Autodesk Fusion 360 part; units mm, degrees
sketch "スケッチ1" plane through (0, 0, 0) normal (0, 0, 1) x (1, 0, 0)
  circle A0 centre (0, 0) radius 10.55
  dimension "d1" = 21.1
extrude "押し出し1" add sketch "スケッチ1" along normal blind 2
sketch "スケッチ2" plane through (0, 0, 2) normal (0, 0, 1) x (-1, 0, 0)
  circle A0 centre (0, 0) radius 10.55
  circle A1 centre (0, 0) radius 8.5
  dimension "d4" = 17
extrude "押し出し2" add sketch "スケッチ2" along normal blind 3.2 contours A1
sketch "スケッチ3" plane through (0, 0, 5.2) normal (0, 0, 1) x (-1, 0, 0)
  circle A0 centre (0, 0) radius 8.5
  circle A1 centre (0, 0) radius 10.55
extrude "押し出し3" add sketch "スケッチ3" along normal blind 2 contours A0 | A1
sketch "スケッチ4" plane through (0, 0, 7.2) normal (0, 0, 1) x (-1, 0, 0)
  line L0 (10.5233, -0.75) -> (-10.5233, -0.75)
  line L1 (10.5233, 0.75) -> (-10.5233, 0.75)
  circle A0 centre (0, 0) radius 10.55
  dimension "d24" = 0.75
  dimension "d25" = 0.75
extrude "押し出し7" add sketch "スケッチ4" along normal blind 30 contours L0 L1 A0
sketch "スケッチ5" plane through (0, -0.75, 0) normal (0, -1, 0) x (1, 0, 0)
  line L0 (-10.4732, 7.2) -> (10.4732, 7.2)
  line L1 (10.5, 7.2) -> (10.5, 37.2)
  line L2 (10.5, 37.2) -> (-10.5, 37.2)
  line L3 (-10.5, 37.2) -> (-10.5, 7.2)
  circle A0 centre (0, 34.2) radius 1.625
  line L4 (0, 34.2) -> (0, 37.2) construction
  line L5 (10.4732, 7.2) -> (10.5, 7.2)
  line L6 (-10.5, 7.2) -> (-10.4732, 7.2)
  line L7 (-10.5233, 7.2) -> (10.5233, 7.2)
  line L8 (10.5233, 7.2) -> (10.5233, 37.2)
  line L9 (10.5233, 37.2) -> (-10.5233, 37.2)
  line L10 (-10.5233, 37.2) -> (-10.5233, 7.2)
  dimension "d13" = 3.25
  dimension "d14" = 3
extrude "押し出し8" cut sketch "スケッチ5" against normal up to surface (1.5 mm away) contours A0
sketch "スケッチ8" plane through (0, 0, 7.2) normal (0, 0, 1) x (-1, 0, 0)
  line L0 (-10.5233, 0.75) -> (10.5233, 0.75)
  arc A0 (10.5233, 0.75) -> (-10.5233, 0.75) centre (0, 0) ccw
  line L1 (0.75, -10.5233) -> (0.75, 10.5233)
  line L2 (-0.75, -10.5233) -> (-0.75, 10.5233)
  arc A1 (-10.5233, -0.75) -> (10.5233, -0.75) centre (0, 0) ccw
  dimension "d30" = 0.75
  dimension "d31" = 0.75
extrude "押し出し9" add sketch "スケッチ8" along normal blind 20 contours L0 A0 L1 L2 | L0 L1 L2 A1
Work out the finished part from the listing and answer in its coordinate system (mm). A direction names the side the tool comes from. Coordinates: 2 decimals unless noted, no trailing zeros. Order: outer loops, then holes, each group sorted by start corner. A loop starts at its lowest first (then second) coordinate and runs counter-clockwise, first axis right, second up. Notation, with made-up numbers: (38, -1) - (92, -1) arc R22 ccw to (92, 36) - close; hole circle Ø3 at (12.25, -13). An arc over 180 degrees is marked (long way). Put each result on its own line as item: value. Start each with the question number.
1) Find section C-C (y = 0). Give the vertices of the cut face in (x, z) (3 decimals), plus the area to 3 significant figures.
2) Find section A-A (z = 34.2). Give the vertices of the cut face in (x, y) (3 decimals), plus the area to 3 significant figures.
3) For faces 4 (the flat face through (-4, 4, 7.2)), 5 (the flat face through (-1, -9, 5.2)), 6 (the flat face through (-4, -5, 7.2)), 7 (the flat face through (0.75, 6, 17)), determine the directions among +Z, -Z, +X, -X, +Y, -Y from which every point of the face is accessible in a straight line to the end or side of a thin tool.
4) Find the intervals of material crossed by line 1 (Z direction, x = 9, y = -4); line 2 (Y direction, x = 0.25, z = 5); line 3 (Z direction, x = 0, y = 0.4) (3 decimals), in increasing order. Write a range as from..to.
5) For a pull along Z with two mould halves and no side action, classify faces 1 (the flat face through (1, 9, 2)), 2 (the flat face through (2, -0.75, 22)), 3 (the flat face through (0, 0, 0)) as released by +Z, released by -Z, zero draft, split by the parting line, or undercut.
6) Flat-ended cylindrical pins translate along their axes: pin 1 (3 mm diameter, centred on x = -8, y = 3, fed in from +Z); pin 2 (8 mm diameter, centred on x = 5, y = -4.5, fed in from +Z); pin 3 (1.7 mm diameter, centred on x = -0.5, y = -7.5, fed in from +Z); pin 4 (3 mm diameter, centred on y = 8.5, z = 6, fed in from -X). Find the tip coordinate at first contact, or state that the pin passes through.
7) Find section D-D (z = 18.5). Give the vertices of the cut face in (x, y).
8) Find section B-B (x = 0). Give the vertices of the cut face in (y, z) (3 decimals), plus the area to 3 significant figures.
Results list:
1. outline: (-10.55, 0) - (10.55, 0) - (10.55, 2) - (8.5, 2) - (8.5, 5.2) - (10.55, 5.2) - (10.55, 37.2) - (-10.55, 37.2) - (-10.55, 5.2) - (-8.5, 5.2) - (-8.5, 2) - (-10.55, 2) - close; hole circle Ø3.25 at (0, 34.2)
1. area: 764 mm^2
2. outline: (-10.523, -0.75) - (-1.625, -0.75) - (-1.625, 0.75) - (-10.523, 0.75) arc R10.55 ccw to start; (1.625, -0.75) - (10.523, -0.75) arc R10.55 ccw to (10.523, 0.75) - (1.625, 0.75) - close
2. area: 26.7 mm^2
3. face 4: +Z, -X, +Y
3. face 5: none
3. face 6: +Z, -X, -Y
3. face 7: +Z, +X, +Y
4. line 1: z = 0..2, 5.2..7.2
4. line 2: y = -8.5..8.5
4. line 3: z = 0..32.575, 35.825..37.2
5. face 1: undercut
5. face 2: zero draft
5. face 3: released by -Z
6. pin 1: stops at z = 7.2
6. pin 2: stops at z = 37.2
6. pin 3: stops at z = 27.2
6. pin 4: stops at x = -7.89
7. outline: (-10.52, -0.75) - (-0.75, -0.75) - (-0.75, -10.52) arc R10.55 ccw to (0.75, -10.52) - (0.75, -0.75) - (10.52, -0.75) arc R10.55 ccw to (10.52, 0.75) - (0.75, 0.75) - (0.75, 10.52) arc R10.55 ccw to (-0.75, 10.52) - (-0.75, 0.75) - (-10.52, 0.75) arc R10.55 ccw to start
8. outline: (-10.55, 0) - (10.55, 0) - (10.55, 2) - (8.5, 2) - (8.5, 5.2) - (10.55, 5.2) - (10.55, 27.2) - (0.75, 27.2) - (0.75, 32.575) - (-0.75, 32.575) - (-0.75, 27.2) - (-10.55, 27.2) - (-10.55, 5.2) - (-8.5, 5.2) - (-8.5, 2) - (-10.55, 2) - close; (-0.75, 35.825) - (0.75, 35.825) - (0.75, 37.2) - (-0.75, 37.2) - close
8. area: 571 mm^2
